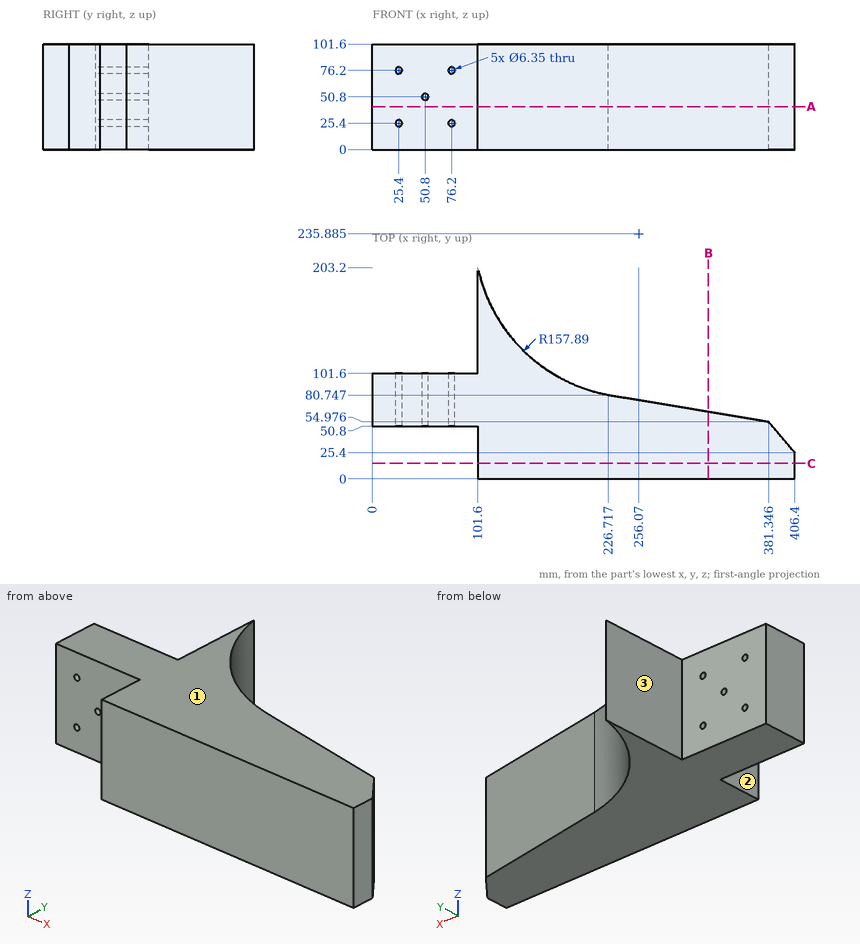
Verification items for this drawing (mm, ordinates from the low corner). A direction names the side the tool comes from. Give positions to 0.01 mm unless a question says otherwise; leave off trailing zeros. Order: outer loops, then holes, each group sorted by start corner. A loop starts at its lowest first (then second) coordinate and runs counter-clockwise, first axis right, second up. Notation, with made-up numbers: M 68.25,55.25 L 125.25,55.25 A26 ccw 125.25,92.25 Z; hole C 30.25,58 d10. An arc over 180 degrees is marked long. Use a Markdown table: item, result.
Item 1: Tool access check on the marked faces 1, 2 and 3. Record the directions out of +Z, -Z, +X, -X, +Y, -Y that give a thin tool (end or side, any length) a straight path to the whole face; none if there is none.
Answers follow:
| item | result |
|---|---|
| face 1 | +Z, +X, -X, +Y, -Y |
| face 2 | +Z, -Z, -X, -Y |
| face 3 | +Z, -Z, -X, +Y |
Item 2: Depth check by flat-ended pin: P1, Ø7.5, axis at x = 50.8, z = 50.8, coming from the -Y side; P2, Ø10, axis at x = 25.4, z = 76.2, coming from the +Y side; P3, Ø2, axis at y = 48, z = 17.5, coming from the +X side. Enter the tip coordinate at first touch or a pass-through.
Answers follow:
| item | result |
|---|---|
| P1 | stops at y = 50.8 |
| P2 | stops at y = 101.6 |
| P3 | stops at x = 388.1 |
Item 3: Section check B-B (x = 323). Record the cut outline in (y, z), and give its area (3 significant figures).
Answers follow:
| item | result |
|---|---|
| outline | M 0,0 L 64.7,0 L 64.7,101.6 L 0,101.6 Z |
| area | 6,570 mm2 |
Item 4: Section check C-C (y = 15). Record the cut outline in (x, z), and give its area (3 significant figures).
Answers follow:
| item | result |
|---|---|
| outline | M 101.6,0 L 406.4,0 L 406.4,101.6 L 101.6,101.6 Z |
| area | 31,000 mm2 |
Item 5: Section check A-A (z = 41.5). Record the cut outline in (x, y) (1 decimal).
Answers follow:
| item | result |
|---|---|
| outline | M 0,50.8 L 101.6,50.8 L 101.6,0 L 406.4,0 L 406.4,25.4 L 381.3,55 L 226.7,80.7 A157.9 cw 101.6,203.2 L 101.6,101.6 L 0,101.6 Z |
Item 6: Material ranges on line 1 along Z through (x, y) = (25.4, 62) (1 decimal); line 2 along Z through (x, y) = (50.8, 79.5) (1 decimal); line 3 along Y through (x, z) = (69, 71), recorded low to high.
Answers follow:
| item | result |
|---|---|
| line 1 | z = 0 to 22.2, 28.6 to 73, 79.4 to 101.6 |
| line 2 | z = 0 to 47.6, 54 to 101.6 |
| line 3 | y = 50.8 to 101.6 |
